The listing builds one solid part. Answer for the finished solid, in the listing's coordinates (mm). A direction names the side the tool comes from. Round coordinates to 2 decimals unless told otherwise and drop trailing zeros. Write each loop counter-clockwise with the first axis right and the second up, starting at its lowest first coordinate (ties: lowest second). Pieces come first, ordered by that corner, then holes. Notation, with made-up numbers: M -39.75,57.5 L -11.75,57.5 A14 cw -11.75,68.5 Z; hole C 25,15.25 d3. An arc over 180 degrees is marked long. One line per item, written item: value. Start each with the question number.
(1) Consider probe 1 along Y at (x, z) = (8, 0); probe 2 along X at (y, z) = (-3, -3.5); probe 3 along Y at (x, z) = (12.5, 0.5). Determine where each line is inside the solid, lowest interval first.
(2) For a pull along Z with two mould halves and no side action, classify faces 1 (the flat face through (-1, -1, -0.5)), 2 (the cylindrical face through (14, -2, 0)) as released by +Z, released by -Z, zero draft, split by the parting line, or undercut.
(3) For faces 3 (the cylindrical face through (4.242, 0.541, 1.717)), 4 (the conical face through (26, 0, -1)), 5 (the flat face through (-0.146, -0.007, -1.514)), determine the directions among +Z, -Z, +X, -X, +Y, -Y from which every point of the face is accessible in a straight line to the end or side of a thin tool.
(4) Section B-B (x = 4) is taken. Determine the outline of the cut face in (y, z).
(5) Given P1, Ø2, axis at y = 0, z = 2, coming from the -X side; P2, Ø3, axis at x = 18, y = 3, coming from the +Z side; P3, Ø2, axis at x = 0, z = 2, coming from the -Y side, each flat-ended and moving along its own axis, determine where each tip first touches the part or whether it passes through.
(6) Section A-A (x = 15.75) is taken. Determine the outline of the cut face in (y, z).
```python
from build123d import *

# Parameters (mm, degrees)
F3_DEPTH = 0.5


# Not quite as in the source:
# - a pattern or mirror of a feature is missing from the dataset's text; its kind, count and spacing are read off the source's solid


with BuildPart() as f1:
    # F0 (on Front) → F1 (revolve)
    with BuildSketch(Plane.XZ):
        with BuildLine():
            Line((28, 0), (24, 2))
            Line((24, 2), (5, 2))
            Line((5, 2), (4.8, 1.8))
            Line((4.8, 1.8), (3.7, 1.8))
            Line((3.7, 1.8), (0, 5.5))
            Line((0, 5.5), (-0.3, 5.5))
            ThreePointArc((-0.3, 5.5), (-1.196512283, 2.814693589), (-1.5, 0))
            Line((-1.5, 0), (28, 0))
        make_face()
    revolve(axis=Axis((13.25, 0, 0), (-1, 0, 0)))

    # F2 (on Front) → F3 (cut, symmetric)
    with BuildSketch(Plane.XZ):
        Polygon((-1.2611724095, 2.5), (-1.5, 2.5), (-1.5, 0), (-1.5, -2.5), (-1.2611724095, -2.5), (1, -0.5), (1, 0), (1, 0.5), align=None)
    f3 = extrude(amount=F3_DEPTH, both=True, mode=Mode.SUBTRACT)

    # F3_copies: F3 across plane
    add(f3.mirror(Plane(origin=(0, 0, 0), x_dir=(0, 0.7071067832, 0.7071067792), z_dir=(4.5e-09, -0.7071067792, 0.7071067832))), mode=Mode.SUBTRACT)


solid = f1.part
```
Recorded:
1. probe 1: y = -2 to 2
1. probe 2: x = -0.67 to 0.89
1. probe 3: y = -1.94 to 1.94
2. face 1: undercut
2. face 2: split by the parting line
3. face 3: none
3. face 4: +X
3. face 5: -X
4. outline: C 0,0 d3.6
5. P1: stops at x = -1.44
5. P2: stops at z = 1.32
5. P3: stops at y = -5.41
6. outline: C 0,0 d4
